Autodesk Inventor part; units mm, degrees
ref_plane "YZ Plane" through (0, 0, 0) normal (1, 0, 0) x (0, 1, 0)
ref_plane "XZ Plane" through (0, 0, 0) normal (0, 1, 0) x (-1, 0, 0)
ref_plane "XY Plane" through (0, 0, 0) normal (0, 0, 1) x (1, 0, 0)
sketch "Sketch1" plane through (0, 0, 0) normal (0, 1, 0) x (-1, 0, 0)
  line L0 (-19.95, 199) -> (19.95, 199)
  line L1 (19.95, 199) -> (19.95, -199)
  line L2 (19.95, -199) -> (-19.95, -199)
  line L3 (-19.95, -199) -> (-19.95, 199)
  line L4 (-19.95, 199) -> (19.95, -199) construction
  line L5 (19.95, 199) -> (-19.95, -199) construction
  point P0 (0, 0)
  dimension "d0" = 39.9
  dimension "d1" = 398
extrude "Extrusion1" add sketch "Sketch1" along normal mid plane 21
sketch "Sketch2" plane through (0, 10.5, 0) normal (0, 1, 0) x (1, 0, 0)
  line L0 (-19.95, -199) -> (19.95, -199)
  line L1 (19.95, 199) -> (-19.95, 199)
  line L2 (-11.95, -199) -> (-7.95, -199)
  line L3 (-7.95, -199) -> (-7.95, 199)
  line L4 (-7.95, 199) -> (-11.95, 199)
  line L5 (-11.95, 199) -> (-11.95, -199)
  line L6 (0, -199) -> (0, 199) construction
  line L7 (-19.95, 199) -> (-19.95, -199)
  line L8 (7.95, -199) -> (11.95, -199)
  line L9 (11.95, -199) -> (11.95, 199)
  line L10 (11.95, 199) -> (7.95, 199)
  line L11 (7.95, 199) -> (7.95, -199)
  point P0 (0, 0)
  point P1 (-11.95, 199)
  dimension "d4" = 4
  dimension "d5" = 8
extrude "Extrusion2" cut sketch "Sketch2" against normal blind 5 contours L5 L1 L3 L0 | L11 L1 L9 L0
mirror "Mirror1" about plane through (0, 0, 0) normal (0, 1, 0) of "Extrusion2"
properties part number "Linear Rail Base"
Input: part model. Units: mm. Frame: model coordinates. Coordinates: 2 decimals unless noted, no trailing zeros. Loops run counter-clockwise (first coordinate to the right, second up) from the corner with the lowest first, then second, coordinate; pieces in that order, holes last. Notation, with made-up numbers: (17.25, -10) - (57.25, -10) arc R14 ccw to (57.25, 16) - close; hole circle Ø4 at (10.25, -4.75). An arc over 180 degrees is marked (long way). Answer in a Markdown table with one row per item. Add a question column.
Item 1: Contact query for flat-ended pins moving along their axis: P1, Ø2, axis at x = -9, z = 5, coming from the +Y side; P2, Ø1.2, axis at x = 9.5, z = -11, coming from the -Y side. Output: stop coordinate, or through.
Item 2: Section query A-A on z = 6.5. Return the cut outline in (x, y).
Item 3: Line query: line 1 along X through (y, z) = (-6, -130); line 2 along Y through (x, z) = (11, -115.5). Output: solid intervals per line, ascending. Write a range as [from, to].
Recorded:
| question | item | result |
|---|---|---|
| 1 | P1 | y = 5.5 |
| 1 | P2 | y = -5.5 |
| 2 | outline | (-19.95, -10.5) - (-11.95, -10.5) - (-11.95, -5.5) - (-7.95, -5.5) - (-7.95, -10.5) - (7.95, -10.5) - (7.95, -5.5) - (11.95, -5.5) - (11.95, -10.5) - (19.95, -10.5) - (19.95, 10.5) - (11.95, 10.5) - (11.95, 5.5) - (7.95, 5.5) - (7.95, 10.5) - (-7.95, 10.5) - (-7.95, 5.5) - (-11.95, 5.5) - (-11.95, 10.5) - (-19.95, 10.5) - close |
| 3 | line 1 | [-19.95, -11.95], [-7.95, 7.95], [11.95, 19.95] |
| 3 | line 2 | [-5.5, 5.5] |
